Can you work these out from the model? Positions are in its coordinate system, mm. A direction names the side the tool comes from. Give positions to 0.01 mm unless a question says otherwise; leave off trailing zeros. Loops run counter-clockwise (first coordinate to the right, second up) from the corner with the lowest first, then second, coordinate; pieces in that order, holes last. Notation, with made-up numbers: (30.25, 11) - (70.25, 11) arc R23 ccw to (70.25, 36) - close; hole circle Ø2 at (83.25, 76). An arc over 180 degrees is marked (long way). Answer in a Markdown table with one row per item.
from build123d import *

# Parameters (mm, degrees)
SKETCH1_R           = 4.5
BOSS_EXTRUDE1_DEPTH = 4
FILLET1_R           = 10
CHAMFER2_SIZE       = 1


with BuildPart() as part:
    # Sketch1 → Boss-Extrude1 (new body)
    with BuildSketch(Plane.XY):
        with BuildLine():
            Line((5.984173373, -2.537650299), (33.282244564, 4.776845831))
            Line((33.282244564, 4.776845831), (43.739940984, -1.016288457))
            ThreePointArc((43.739940984, -1.016288457), (55.845872024, -3.149739565), (47.616543526, 5.98170788))
            Line((47.616543526, 5.98170788), (34.332563277, 13.340487326))
            Line((34.332563277, 13.340487326), (3.913621012, 5.189756311))
            ThreePointArc((3.913621012, 5.189756311), (-6.278517871, -1.682323793), (5.984173373, -2.537650299))
        make_face()
        Circle(SKETCH1_R, mode=Mode.SUBTRACT)
        with Locations((50.16, 0)):
            Circle(SKETCH1_R, mode=Mode.SUBTRACT)
    extrude(amount=BOSS_EXTRUDE1_DEPTH)

    # Fillet1
    fillet1_edges = [part.edges().sort_by_distance(p)[0] for p in [
        (33.282244564, 4.776845831, 2),
        (5.984173373, -2.537650299, 2),
        (3.913621012, 5.189756311, 2),
        (34.332563277, 13.340487326, 2),
        (47.616543526, 5.98170788, 2),
        (43.739940984, -1.016288457, 2),
    ]]
    fillet(fillet1_edges, radius=FILLET1_R)

    # Chamfer2
    chamfer2_edges = [part.edges().sort_by_distance(p)[0] for p in [
        (38.699188042, 1.776081634, 0),
        (38.699188042, 1.776081634, 4),
        (19.425508285, 1.063944536, 0),
        (19.425508285, 1.063944536, 4),
        (18.915391461, 9.209468588, 0),
        (18.915391461, 9.209468588, 4),
        (-6.278517871, -1.682323793, 0),
        (41.16264867, 9.55690055, 0),
        (55.845872024, -3.149739565, 0),
        (34.237028938, 12.561560111, 0),
        (41.16264867, 9.55690055, 4),
        (55.845872024, -3.149739565, 4),
        (-6.278517871, -1.682323793, 4),
        (34.237028938, 12.561560111, 4),
        (33.186710225, 3.997918617, 0),
        (33.186710225, 3.997918617, 4),
        (6.91120565, -2.689125301, 0),
        (6.91120565, -2.689125301, 4),
        (47.054714022, 6.734490138, 0),
        (47.054714022, 6.734490138, 4),
        (42.803779737, -0.939245365, 0),
        (42.803779737, -0.939245365, 4),
        (4.640717013, 5.784453649, 0),
        (4.640717013, 5.784453649, 4),
    ]]
    chamfer(chamfer2_edges, length=CHAMFER2_SIZE)


solid = part.part
Q1. Imagine slicing it at C-C, the plane x = 20. Write out the boundary of the cut face in (y, z), and give its area (3 significant figures).
Checked values:
| item | result |
|---|---|
| outline | (1.22, 1) - (2.25, 0) - (8.46, 0) - (9.5, 1) - (9.5, 3) - (8.46, 4) - (2.25, 4) - (1.22, 3) - close |
| area | 31.1 mm² |
Q2. If I drill on line 1 (Y direction, x = 50.16, z = 2.4); line 2 (Y direction, x = 49, z = 3); line 3 (X direction, y = -4.75, z = 2.3), over which ranges is the centre line in solid material (lowest first)? Write a range as [from, to].
Checked values:
| item | result |
|---|---|
| line 1 | y = [-6.5, -4.5], [4.5, 6.5] |
| line 2 | y = [-6.4, -4.35], [4.35, 6.48] |
| line 3 | x = [-4.44, 4.44], [45.72, 54.6] |
Q3. On a 3-axis mill with a long thin cutter (end or side, diameter ignored), from which of +Z, -Z, +X, -X, +Y, -Y can I reach the whole of each face in a straight line? I mean faces 4 (the face through (41.21, 9.53, 1.99)), 5 (the face through (6.94, -2.67, 2.01)), 6 (the face through (38.91, 2.22, 3.49)), 7 (the face through (19.16, 1.5, 0.51)). Say none if no direction works.
Checked values:
| item | result |
|---|---|
| face 4 | +Z, -Z, +X, +Y |
| face 5 | +Z, -Z, -Y |
| face 6 | +Z, -Y |
| face 7 | -Z, -Y |
Q4. For pin 1 (6 mm diameter, centred on x = 28.5, y = -0.5, fed in from -Z); pin 2 (10.5 mm diameter, centred on x = 50.16, y = 0, fed in from -Z); pin 3 (2 mm diameter, centred on y = 7, z = 1.5, fed in from +X); pin 4 (1.5 mm diameter, centred on x = 38.5, z = 3.5, fed in from -Y), each with a flat end and sliding along its axis, tell me the tip position at first contact or that it passes through.
Checked values:
| item | result |
|---|---|
| pin 1 | passes through |
| pin 2 | stops at z = 0 |
| pin 3 | stops at x = 52.66 |
| pin 4 | stops at y = 1.58 |
Q5. Imagine slicing it at D-D, the plane y = 2.25. Count the separate pieces of the cut face and the enclosed holes in it, and give its area (3 significant figures).
Checked values:
| item | result |
|---|---|
| separate pieces | 4 |
| enclosed holes | 0 |
| area | 123 mm² |
Q6. Imagine slicing it at B-B, the plane z = 1.95. Write out the boundary of the cut face in (x, y).
Checked values:
| item | result |
|---|---|
| outline | (1.9, 6.22) arc R6.5 ccw (long way) to (4.75, -4.44) arc R10 cw to (9.47, -1.6) - (29.38, 3.73) arc R10 cw to (36.82, 2.82) - (40.58, 0.73) arc R10 cw to (44.48, -3.16) arc R6.5 ccw (long way) to (49.82, 6.49) arc R10 cw to (44.46, 7.73) - (37.87, 11.38) arc R10 ccw to (30.43, 12.3) - (7.4, 6.12) arc R10 cw to start; hole circle Ø9 at (0, 0); hole circle Ø9 at (50.16, 0) |
Q7. Imagine slicing it at A-A, the plane x = 0. Write out the boundary of the cut face in (y, z), and give its area (3 significant figures).
Checked values:
| item | result |
|---|---|
| outline | (-6.5, 1) - (-5.5, 0) - (-4.5, 0) - (-4.5, 4) - (-5.5, 4) - (-6.5, 3) - close; (4.5, 0) - (5.5, 0) - (6.5, 1) - (6.5, 3) - (5.5, 4) - (4.5, 4) - close |
| area | 14.0 mm² |
Q8. If we mould it in two halves opening along Y, with no side actions, what happens to faces 1 (the face through (25, 4, 0)), 2 (the face through (45.664, 0.198, 1.972)), 3 (the face through (55.75, -3.32, 1.99))? For each: released by +Y, released by -Y, zero draft, split by the parting line, or undercut.
Checked values:
| item | result |
|---|---|
| face 1 | zero draft |
| face 2 | undercut |
| face 3 | split by the parting line |
